from build123d import *

# Parameters (mm, degrees)
SKETCH_1_R          = 1.35
SKETCH_1_R_2        = 1
SKETCH_1_R_3        = 1.25
EXTRUDE_1_DEPTH     = 2
FILLET_1_R          = 3
SKETCH_3_W          = 12.7
SKETCH_3_H          = 30.365325547
SKETCH_3_W_2        = 13
SKETCH_3_H_2        = 34.884674453
SKETCH_3_W_3        = 42.4
SKETCH_3_H_3        = 8.100647313
SKETCH_3_H_4        = 8.099352903
CUT_EXTRUDE_1_DEPTH = 60.74330897
FILLET_2_R          = 3
FILLET_3_R          = 1.5
CHAMFER_1_SIZE      = 1.5


with BuildPart() as part:
    # 草图1 → 凸台-拉伸1 (new body)
    with BuildSketch(Plane(origin=(0, 0, 0), x_dir=(1, 0, 0), z_dir=(0, 1, 0))):
        with BuildLine():
            Line((-29.7, -30.13671529), (-29.7, -43.600647313))
            Line((-29.7, -43.600647313), (29.7, -43.600647313))
            Line((29.7, -43.600647313), (29.7, -30.13671529))
            ThreePointArc((29.7, -30.13671529), (29.446106374, -29.2429724), (28.760263112, -28.616189066))
            Line((28.760263112, -28.616189066), (24.97140873, -26.721761875))
            ThreePointArc((24.97140873, -26.721761875), (24.043503141, -25.873760893), (23.7, -24.664579335))
            Line((23.7, -24.664579335), (23.7, 32.86328471))
            ThreePointArc((23.7, 32.86328471), (24.043503141, 34.072466267), (24.97140873, 34.920467249))
            Line((24.97140873, 34.920467249), (28.760263112, 36.81489444))
            ThreePointArc((28.760263112, 36.81489444), (29.446106374, 37.441677774), (29.7, 38.335420665))
            Line((29.7, 38.335420665), (29.7, 41.863284896))
            ThreePointArc((29.7, 41.863284896), (29.446106374, 42.757027787), (28.760263112, 43.383811121))
            Line((28.760263112, 43.383811121), (24.971408673, 45.278238341))
            ThreePointArc((24.971408673, 45.278238341), (24.043503084, 46.126239322), (23.699999943, 47.33542088))
            Line((23.699999943, 47.33542088), (23.699999943, 48.899352903))
            ThreePointArc((23.699999943, 48.899352903), (22.850609608, 50.949962568), (20.799999943, 51.799352902))
            Line((20.799999943, 51.799352902), (17.526051986, 51.799352902))
            Line((17.526051986, 51.799352902), (13.526051986, 51.099352903))
            Line((13.526051986, 51.099352903), (-13.5260521, 51.099352903))
            Line((-13.5260521, 51.099352903), (-17.5260521, 51.799352903))
            Line((-17.5260521, 51.799352903), (-20.800000057, 51.799352903))
            ThreePointArc((-20.800000057, 51.799352903), (-22.850609723, 50.949962568), (-23.700000057, 48.899352903))
            Line((-23.700000057, 48.899352903), (-23.700000057, 47.33542088))
            ThreePointArc((-23.700000057, 47.33542088), (-24.043503184, 46.126239345), (-24.97140874, 45.278238364))
            Line((-24.97140874, 45.278238364), (-28.760263161, 43.383811045))
            ThreePointArc((-28.760263161, 43.383811045), (-29.446106456, 42.757027659), (-29.700000093, 41.86328471))
            Line((-29.700000093, 41.86328471), (-29.700000093, 38.335420665))
            ThreePointArc((-29.700000093, 38.335420665), (-29.446106448, 37.44167771), (-28.760263093, 36.814894415))
            Line((-28.760263093, 36.814894415), (-24.971408738, 34.920467256))
            ThreePointArc((-24.971408738, 34.920467256), (-24.043503143, 34.072466274), (-23.7, 32.863284713))
            Line((-23.7, 32.863284713), (-23.7, -24.664579335))
            ThreePointArc((-23.7, -24.664579335), (-24.043503141, -25.873760893), (-24.97140873, -26.721761875))
            Line((-24.97140873, -26.721761875), (-28.760263112, -28.616189066))
            ThreePointArc((-28.760263112, -28.616189066), (-29.446106374, -29.2429724), (-29.7, -30.13671529))
        make_face()
        with Locations(Location((-27, 40, 0), (0, 0, 270))):
            Circle(SKETCH_1_R, mode=Mode.SUBTRACT)
        with Locations(Location((27, 40, 0), (0, 0, 270))):
            Circle(SKETCH_1_R, mode=Mode.SUBTRACT)
        with Locations(Location((-27, -40, 0), (0, 0, 270))):
            Circle(SKETCH_1_R_2, mode=Mode.SUBTRACT)
        with Locations(Location((26.5, -38.5, 0), (0, 0, 270))):
            Circle(SKETCH_1_R_2, mode=Mode.SUBTRACT)
        with Locations(Location((-27, -32, 0), (0, 0, 270))):
            Circle(SKETCH_1_R_3, mode=Mode.SUBTRACT)
        with Locations(Location((27, -32, 0), (0, 0, 270))):
            Circle(SKETCH_1_R_3, mode=Mode.SUBTRACT)
    extrude(amount=EXTRUDE_1_DEPTH)

    # 圆角1
    fillet_1_edges = [part.edges().sort_by_distance(p)[0] for p in [
        (29.7, 1, 43.600647313),
        (-29.7, 1, 43.600647313),
    ]]
    fillet(fillet_1_edges, radius=FILLET_1_R)

    # 草图3 → 切除-拉伸1 (cut, through all)
    with BuildSketch(Plane(origin=(0, 2, 0), x_dir=(1, 0, 0), z_dir=(0, 1, 0))):
        with Locations((14.85, -13.817337227)):
            Rectangle(SKETCH_3_W, SKETCH_3_H)
        with Locations((0, -13.817337227)):
            Rectangle(SKETCH_3_W_2, SKETCH_3_H)
        with Locations((-14.85, 21.307662773)):
            Rectangle(SKETCH_3_W, SKETCH_3_H_2)
        with Locations((0, 21.307662773)):
            Rectangle(SKETCH_3_W_2, SKETCH_3_H_2)
        with Locations((-14.85, -13.817337227)):
            Rectangle(SKETCH_3_W, SKETCH_3_H)
        with Locations((14.85, 21.307662773)):
            Rectangle(SKETCH_3_W, SKETCH_3_H_2)
        with Locations((0, -36.550323656)):
            Rectangle(SKETCH_3_W_3, SKETCH_3_H_3)
        with Locations((0, 45.549676452)):
            Rectangle(SKETCH_3_W_3, SKETCH_3_H_4)
    extrude(amount=-CUT_EXTRUDE_1_DEPTH, mode=Mode.SUBTRACT)

    # 圆角2
    fillet_2_edges = [part.edges().sort_by_distance(p)[0] for p in [
        (21.2, 1, -1.365325547),
        (21.2, 1, 29),
        (8.5, 1, 29),
        (8.5, 1, -1.365325547),
        (-21.2, 1, 29),
        (-21.2, 1, -1.365325547),
        (-8.5, 1, -1.365325547),
        (-8.5, 1, 29),
        (-6.5, 1, 29),
        (-6.5, 1, -1.365325547),
        (6.5, 1, -1.365325547),
        (6.5, 1, 29),
        (-6.5, 1, -3.865325547),
        (-6.5, 1, -38.75),
        (6.5, 1, -38.75),
        (6.5, 1, -3.865325547),
        (21.2, 1, -38.75),
        (21.2, 1, -3.865325547),
        (8.5, 1, -3.865325547),
        (8.5, 1, -38.75),
        (-21.2, 1, -3.865325547),
        (-21.2, 1, -38.75),
        (-8.5, 1, -38.75),
        (-8.5, 1, -3.865325547),
    ]]
    fillet(fillet_2_edges, radius=FILLET_2_R)

    # 圆角3
    fillet_3_edges = [part.edges().sort_by_distance(p)[0] for p in [
        (-21.2, 1, 40.600647313),
        (-21.2, 1, 32.5),
        (21.2, 1, 32.5),
        (21.2, 1, 40.600647313),
        (-21.2, 1, -41.5),
        (-21.2, 1, -49.599352903),
        (21.2, 1, -49.599352903),
        (21.2, 1, -41.5),
    ]]
    fillet(fillet_3_edges, radius=FILLET_3_R)

    # 倒角1
    chamfer_1_edges = [part.edges().sort_by_distance(p)[0] for p in [
        (-27, 2, 39),
        (26.5, 2, 37.5),
    ]]
    chamfer(chamfer_1_edges, length=CHAMFER_1_SIZE)


solid = part.part
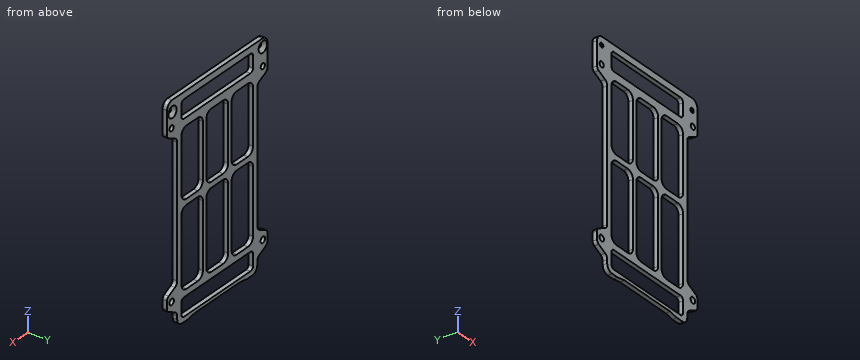
Check sheet for the modelled part. Datum: model origin and axes. Units: mm. Round coordinates to 2 decimals unless told otherwise and drop trailing zeros. Order: outer loops, then holes, each group sorted by start corner. A loop starts at its lowest first (then second) coordinate and runs counter-clockwise, first axis right, second up. Notation, with made-up numbers: M 24.5,-29.5 L 83.5,-29.5 A16 ccw 83.5,-16.5 Z; hole C 33.5,-17.5 d10. An arc over 180 degrees is marked long. One line per item, written item: value. Start each with the question number.
1. Scan lines: line 1 along X through (y, z) = (1.4, -29.5); line 2 along X through (y, z) = (0.6, -40); line 3 along X through (y, z) = (1, 34.5). Record each from-to range of solid material in increasing order.
2. Section check A-A on z = 23. Enter the section's corners in (x, y).
3. Section check C-C on x = 15. Enter the section's corners in (y, z), and give its area (3 significant figures).
4. Gauge pin test, flat ends, axial feed: P1, Ø1, axis at x = 1.5, y = 1, coming from the -Z side; P2, Ø1, axis at y = 1.5, z = -17.5, coming from the +X side; P3, Ø6, axis at x = 10.5, z = -15.5, coming from the +Y side; P4, Ø2, axis at x = -27, z = -40, coming from the +Y side. Record the tip position at first contact, or that the pin passes through.
5. Section check D-D on y = 1.3. Give the number of separate pieces and of enclosed holes in the cut face, and give its area (3 significant figures).
6. Section check B-B on z = -40. Enter the section's corners in (x, y).
Results found:
1. line 1: -23.7 to -21.2, -8.5 to -6.5, 6.5 to 8.5, 21.2 to 23.7
1. line 2: -29.7 to -28.35, -25.65 to 25.65, 28.35 to 29.7
1. line 3: -29.7 to -21.2, 21.2 to 29.7
2. outline: M -23.7,0 L -21.2,0 L -21.2,2 L -23.7,2 Z; M -8.5,0 L -6.5,0 L -6.5,2 L -8.5,2 Z; M 6.5,0 L 8.5,0 L 8.5,2 L 6.5,2 Z; M 21.2,0 L 23.7,0 L 23.7,2 L 21.2,2 Z
3. outline: M 0,-51.36 L 2,-51.36 L 2,-49.6 L 0,-49.6 Z; M 0,-41.5 L 2,-41.5 L 2,-38.75 L 0,-38.75 Z; M 0,-3.87 L 2,-3.87 L 2,-1.37 L 0,-1.37 Z; M 0,29 L 2,29 L 2,32.5 L 0,32.5 Z; M 0,40.6 L 2,40.6 L 2,43.6 L 0,43.6 Z
3. area: 27.0 mm^2
4. P1: z = -51.1
4. P2: x = 23.7
4. P3: y = 2
4. P4: through
5. separate pieces: 1
5. enclosed holes: 14
5. area: 1,610 mm^2
6. outline: M -29.7,0 L -28.35,0 L -28.35,2 L -29.7,2 Z; M -25.65,0 L 25.65,0 L 25.65,2 L -25.65,2 Z; M 28.35,0 L 29.7,0 L 29.7,2 L 28.35,2 Z
